from build123d import *

# Parameters (mm, degrees)
SKETCH1_R           = 10
BOSS_EXTRUDE1_DEPTH = 600
SKETCH2_R           = 10
BOSS_EXTRUDE2_DEPTH = 22.5


with BuildPart() as part:
    # Sketch1 → Boss-Extrude1 (new body)
    with BuildSketch(Plane.XY):
        Circle(SKETCH1_R)
        Polygon((7.665529004, -0.706345771), (4.444477884, 6.285369965), (-3.22105112, 6.991715737), (-7.665529004, 0.706345771), (-4.444477884, -6.285369965), (3.22105112, -6.991715737), align=None, mode=Mode.SUBTRACT)
    extrude(amount=BOSS_EXTRUDE1_DEPTH)

    # Sketch2 → Boss-Extrude2 (add)
    with BuildSketch(Plane.XY):
        Circle(SKETCH2_R)
    extrude(amount=-BOSS_EXTRUDE2_DEPTH)


solid = part.part
For this review, take the finished solid that the model builds, in its own axes (mm). Round coordinates to 2 decimals unless told otherwise and drop trailing zeros. Loops run counter-clockwise (first coordinate to the right, second up) from the corner with the lowest first, then second, coordinate; pieces in that order, holes last. Notation, with made-up numbers: (28.25, -31) - (70.25, -31) arc R29 cw to (70.25, -8) - close; hole circle Ø1 at (49.5, 63.25). An arc over 180 degrees is marked (long way). One line per question, with ' | ' between items.
Q1. Take a section at B-B (x = 0). Give the boundary of the cut face in (y, z).
Taken from the geometry:
outline: (-10, -22.5) - (10, -22.5) - (10, 600) - (6.69, 600) - (6.69, 0) - (-6.69, 0) - (-6.69, 600) - (-10, 600) - close
Q2. The part is to be moulded in two halves that separate along Y. For faces 1 (the cylindrical face through (-2.17, -9.76, 293.11)), 2 (the flat face through (0, 0, -22.5)), 3 (the flat face through (0, 0, 0)), say which applies: released by +Y, released by -Y, zero draft, split by the parting line, or undercut.
Taken from the geometry:
face 1: split by the parting line | face 2: zero draft | face 3: undercut
Q3. Take a section at A-A (z = 439.5). Give the boundary of the cut face in (x, y).
Taken from the geometry:
outline: circle Ø20 at (0, 0); hole (-7.67, 0.71) - (-4.44, -6.29) - (3.22, -6.99) - (7.67, -0.71) - (4.44, 6.29) - (-3.22, 6.99) - close
Q4. For line 1 along X through (y, z) = (0.5, 301); line 2 along Y through (x, z) = (0.25, 281.5); line 3 along Z through (x, y) = (-0.75, 5.25), list the stretches that pass through material, from the lowest coordinate up. Write a range as [from, to].
Taken from the geometry:
line 1: x = [-9.99, -7.57], [7.11, 9.99] | line 2: y = [-10, -6.72], [6.67, 10] | line 3: z = [-22.5, 0]
Q5. For pin 1 (1.5 mm diameter, centred on x = 5.5, z = 415, fed in from +Y); pin 2 (1 mm diameter, centred on x = 3.5, z = 252, fed in from +Y); pin 3 (1 mm diameter, centred on x = -2, z = 284, fed in from +Y), all flat-tipped, find the tip position at first contact; note any pin that passes through.
Taken from the geometry:
pin 1: stops at y = 8.8 | pin 2: stops at y = 9.54 | pin 3: stops at y = 9.89
